Could you check a few things on this model? Use its own coordinates, in mm. Face numbers are marked on the shaded views. A direction names the side the tool comes from. Round coordinates to 2 decimals unless told otherwise and drop trailing zeros. Loops run counter-clockwise (first coordinate to the right, second up) from the corner with the lowest first, then second, coordinate; pieces in that order, holes last.
from build123d import *

# Parameters (mm, degrees)
SKETCH1_W           = 19
SKETCH1_H           = 23.44
SKETCH1_R           = 0.5
BOSS_EXTRUDE1_DEPTH = 1.5
BOSS_EXTRUDE2_DEPTH = 2
FILLET1_R           = 1
SKETCH4_W           = 18.301670477
SKETCH4_H           = 3.380629264
SKETCH4_H_2         = 3.475508354
CUT_EXTRUDE1_DEPTH  = 0.1


with BuildPart() as part:
    # Sketch1 → Boss-Extrude1 (new body)
    with BuildSketch(Plane(origin=(0, 0, 0), x_dir=(1, 0, 0), z_dir=(0, 1, 0))):
        with Locations((9.5, -11.72)):
            Rectangle(SKETCH1_W, SKETCH1_H)
        with Locations((1.88, -1.3)):
            Circle(SKETCH1_R, mode=Mode.SUBTRACT)
        with Locations((4.42, -1.3)):
            Circle(SKETCH1_R, mode=Mode.SUBTRACT)
        with Locations((6.96, -1.3)):
            Circle(SKETCH1_R, mode=Mode.SUBTRACT)
        with Locations((9.5, -1.3)):
            Circle(SKETCH1_R, mode=Mode.SUBTRACT)
        with Locations((12.04, -1.3)):
            Circle(SKETCH1_R, mode=Mode.SUBTRACT)
        with Locations((14.58, -1.3)):
            Circle(SKETCH1_R, mode=Mode.SUBTRACT)
        with Locations((17.12, -1.3)):
            Circle(SKETCH1_R, mode=Mode.SUBTRACT)
    extrude(amount=BOSS_EXTRUDE1_DEPTH)

    # Sketch3 → Boss-Extrude2 (add)
    with BuildSketch(Plane(origin=(0, 1.5, 0), x_dir=(1, 0, 0), z_dir=(0, 1, 0))):
        Polygon((3.832385917, -21.106985825), (3.832385917, -23.44), (15.344727023, -23.44), (15.344727023, -21.106985825), (18.591797592, -21.106985825), (18.591797592, -2.569164761), (0.290127115, -2.569164761), (0.290127115, -21.106985825), align=None)
    extrude(amount=BOSS_EXTRUDE2_DEPTH)

    # Fillet1
    fillet1_edges = [part.edges().sort_by_distance(p)[0] for p in [
        (9.58855647, 3.5, 23.44),
    ]]
    fillet(fillet1_edges, radius=FILLET1_R)

    # Sketch4 → Cut-Extrude1 (cut)
    with BuildSketch(Plane(origin=(0, 3.5, 0), x_dir=(1, 0, 0), z_dir=(0, 1, 0))):
        with Locations((9.440962354, -4.259479393)):
            Rectangle(SKETCH4_W, SKETCH4_H)
        with Locations((9.440962354, -21.702245823)):
            Rectangle(SKETCH4_W, SKETCH4_H_2)
    extrude(amount=-CUT_EXTRUDE1_DEPTH, mode=Mode.SUBTRACT)


solid = part.part
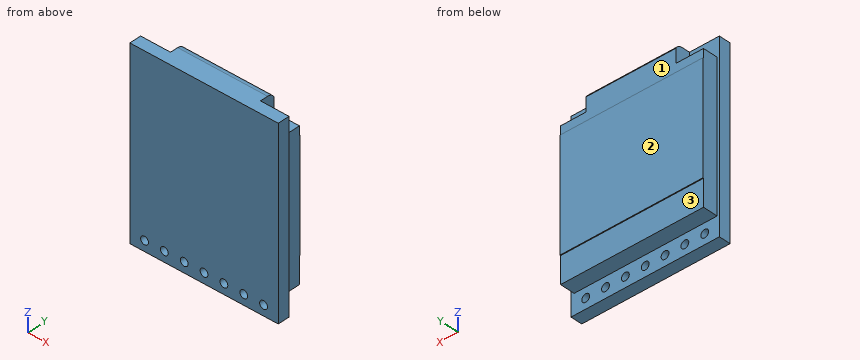
Item 1: If we section it at D-D, the plane y = 2.1: Please give me the cut outline in (x, z).
Results list:
outline: (0.29, 2.57) - (18.59, 2.57) - (18.59, 21.11) - (15.34, 21.11) - (15.34, 23.44) - (3.83, 23.44) - (3.83, 21.11) - (0.29, 21.11) - close
Item 2: If we section it at A-A, the plane x = 17.12: Please give me the cut outline in (y, z).
Results list:
outline: (0, 0) - (1.5, 0) - (1.5, 0.8) - (0, 0.8) - close; (0, 1.8) - (1.5, 1.8) - (1.5, 2.57) - (3.4, 2.57) - (3.4, 5.95) - (3.5, 5.95) - (3.5, 19.96) - (3.4, 19.96) - (3.4, 21.11) - (1.5, 21.11) - (1.5, 23.44) - (0, 23.44) - close
Item 3: If we section it at C-C, the plane x = 3: Please give me the cut outline in (y, z).
Results list:
outline: (0, 0) - (1.5, 0) - (1.5, 2.57) - (3.4, 2.57) - (3.4, 5.95) - (3.5, 5.95) - (3.5, 19.96) - (3.4, 19.96) - (3.4, 21.11) - (1.5, 21.11) - (1.5, 23.44) - (0, 23.44) - close
Item 4: Will these pins go through, and if not, where does the flat tip stop? pin 1 (1.5 mm diameter, centred on y = 2.5, z = 22.5, fed in from +X); pin 2 (1.6 mm diameter, centred on y = 3, z = 10.5, fed in from -X); pin 3 (1.7 mm diameter, centred on x = 11, z = 3.5, fed in from +Y); pin 4 (3 mm diameter, centred on x = 6, z = 21, fed in from +Y).
Results list:
pin 1: stops at x = 15.34
pin 2: stops at x = 0.29
pin 3: stops at y = 3.4
pin 4: stops at y = 3.5
Item 5: For the marked faces 1, 2 and 3, which set-ups out of +Z, -Z, +X, -X, +Y, -Y let a thin tool reach every point of the face, with its end or its side?
Results list:
face 1: +Z, +X, -X, +Y
face 2: +Z, -Z, +X, -X, +Y
face 3: -Z, +X, -X, +Y
Item 6: If we section it at B-B, the plane z = 1.3: Count the separate pieces of the cut face and the enclosed holes in it, then the cut area to 3 significant figures.
Results list:
separate pieces: 8
enclosed holes: 0
area: 18.0 mm2
Item 7: If I drill on line 1 along Z through (x, y) = (1.88, 0.7); line 2 along Z through (x, y) = (2, 2.75); line 3 along Y through (x, z) = (16.75, 5.25), over which ranges is the centre line in solid material (lowest first)?
Results list:
line 1: z = 0 to 0.8, 1.8 to 23.44
line 2: z = 2.57 to 21.11
line 3: y = 0 to 3.4
